Geometry: final body of the model. Coordinates: model frame, mm. A direction names the side the tool comes from. Give positions to 0.01 mm unless a question says otherwise; leave off trailing zeros. Order: outer loops, then holes, each group sorted by start corner. A loop starts at its lowest first (then second) coordinate and runs counter-clockwise, first axis right, second up. Notation, with made-up numbers: (58.25, 3) -> (109.25, 3) arc R21 ccw to (109.25, 20) -> close; hole circle Ø6 at (3.5, 1). An arc over 180 degrees is marked (long way). Write item = value, one per line.
```python
from build123d import *

# Parameters (mm, degrees)
F0_W     = 19.0500004709
F0_H     = 19.05
F0_W_2   = 19.0500002354
F0_W_3   = 19.05
F1_DEPTH = 19.1
F4_DEPTH = 19.05


with BuildPart() as f1:
    # F0 (on Top) → F1 (new body)
    with BuildSketch(Plane.XY):
        with Locations((-28.5750002354, -9.525)):
            Rectangle(F0_W, F0_H)
        with Locations((-9.5250001177, -9.525)):
            Rectangle(F0_W_2, F0_H)
        with Locations((-9.525, -28.575)):
            Rectangle(F0_W_3, F0_H)
    extrude(amount=F1_DEPTH)

    # F3 (on offset) → F4 (join)
    with BuildSketch(Plane.XY.offset(19.05)):
        Polygon((-19.05, 0), (-38.1, 0), (-38.1, -38.1), (0, -38.1), (0, -19.05), (-19.05, -19.05), align=None)
    extrude(amount=F4_DEPTH)


solid = f1.part
```
1) Line query: line 1 (Y direction, x = -4.5, z = 32); line 2 (X direction, y = -20, z = 13). Output: solid intervals per line, ascending. Write a range as from..to.
Check sheet entries:
line_1 = -38.1..-19.05
line_2 = -19.05..0
2) First-contact query: P1, Ø9.5, axis at y = -12, z = 24.5, coming from the +X side; P2, Ø2, axis at y = -30, z = 5, coming from the -X side; P3, Ø9.5, axis at x = -14, y = -7.5, coming from the +Z side. Flat tips, straight axial feed; report the tip coordinate or a pass-through.
Check sheet entries:
P1 = -19.05
P2 = -19.05
P3 = 19.1
3) Section query B-B (x = -6.5). Output: boundary loops of the cut face in (y, z).
Check sheet entries:
outline = (-38.1, 0) -> (0, 0) -> (0, 19.1) -> (-19.05, 19.1) -> (-19.05, 38.1) -> (-38.1, 38.1) -> close
4) Reachability of faces 1 (the face through (0, -24, 15)), 2 (the face through (-19.05, -10, 28)), 3 (the face through (-29, -28, 19.05)) from +Z, -Z, +X, -X, +Y, -Y: full face, straight path, thin tool, end or side. Return the list, or none.
Check sheet entries:
face_1 = +Z, -Z, +X, +Y, -Y
face_2 = +Z, +X, +Y
face_3 = -Z, -X, -Y
5) Section query A-A (y = -23.5). Output: boundary loops of the cut face in (x, z), plus the area to 3 significant figures.
Check sheet entries:
outline = (-38.1, 19.05) -> (-19.05, 19.05) -> (-19.05, 0) -> (0, 0) -> (0, 38.1) -> (-38.1, 38.1) -> close
area = 1,090 mm²
